Geometry check sheet. Reference: the model listing, model coordinates, mm. Face numbers are marked on the shaded views. A direction names the side the tool comes from. Give positions to 0.01 mm unless a question says otherwise; leave off trailing zeros. Loops run counter-clockwise (first coordinate to the right, second up) from the corner with the lowest first, then second, coordinate; pieces in that order, holes last. Notation, with made-up numbers: (80.25, 80) -> (109.25, 80) arc R14 cw to (109.25, 97) -> close; hole circle Ø4 at (-26, 5.25). An arc over 180 degrees is marked (long way). Write each question's results on one line, items separated by ' | '. Start each with the question number.
1) Sectioned sample at B-B on x = -28. Record the cut outline in (y, z).
2) Set-up check for the marked faces 4, 5 and 6: record each of +Z, -Z, +X, -X, +Y, -Y from which the full face is reachable in a straight line by a thin tool's end or side.
3) Draft check along Y on the marked faces 1, 2 and 3. Enter one of: pulls with the +Y half, pulls with the -Y half, needs draft (parallel to the pull), parting line crosses it, or undercut.
4) Scan lines: line 1 (X direction, y = 1, z = 0); line 2 (Y direction, x = -18.5, z = -38); line 3 (Y direction, x = -21.5, z = -37). Record each from-to range of solid material in increasing order. Write a range as from..to.
5) Sectioned sample at D-D on y = -30.5. Record the cut outline in (x, z), then the cut area to 3 significant figures.
6) Sectioned sample at A-A on z = 0. Record the cut outline in (x, y), then the cut area to 3 significant figures.
7) Sectioned sample at C-C on x = 5.08. Record the cut outline in (y, z), then the cut area to 3 significant figures.
8) Depth check by flat-ended pin: pin 1 (5 mm diameter, centred on y = 59, z = -19, fed in from -X); pin 2 (3 mm diameter, centred on y = 13.5, z = -20.5, fed in from +X); pin 3 (1 mm diameter, centred on y = 13, z = -44, fed in from +X). Enter the tip coordinate at first touch or a pass-through.
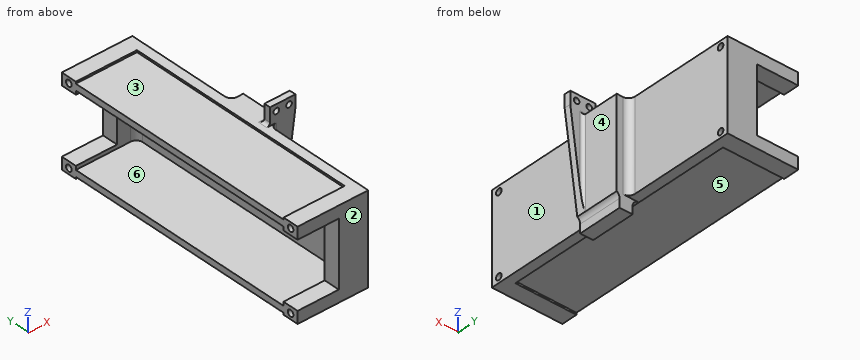
```python
from build123d import *

# Parameters (mm, degrees)
SKETCH1_R           = 1.1303
BOSS_EXTRUDE1_DEPTH = 2.54
SKETCH2_W           = 5.08
SKETCH2_H           = 35.814
BOSS_EXTRUDE2_DEPTH = 15.24
SKETCH3_W           = 35.814
SKETCH3_H           = 106.370628
BOSS_EXTRUDE3_DEPTH = 3.81
FILLET1_R           = 1.27
SKETCH4_W           = 5.191
SKETCH4_H           = 17.78
BOSS_EXTRUDE4_DEPTH = 5.588
SKETCH5_W           = 35.814
SKETCH5_H           = 6.35
BOSS_EXTRUDE5_DEPTH = 7.9756
SKETCH6_W           = 4.826
SKETCH6_H           = 6.35
BOSS_EXTRUDE6_DEPTH = 16.51
BOSS_EXTRUDE8_START = -0.762
SKETCH7_W           = 24.4856
SKETCH7_H           = 93.670628
BOSS_EXTRUDE8_DEPTH = 2.54
FILLET2_R           = 2.54
SKETCH8_R           = 1.27
CUT_EXTRUDE1_DEPTH  = 87.153909833


with BuildPart() as part:
    # Sketch1 → Boss-Extrude1 (new body)
    with BuildSketch(Plane(origin=(0, 0, 0), x_dir=(1, 0, 0), z_dir=(0, 1, 0))):
        Polygon((-2.54, 2.54), (-2.54, 40.132), (2.54, 40.132), (7.62, 2.54), (7.62, -2.54), (-2.54, -2.54), align=None)
        with Locations(Location((0, 0, 0), (0, 0, 270))):
            Circle(SKETCH1_R, mode=Mode.SUBTRACT)
        with Locations(Location((5.08, 0, 0), (0, 0, 270))):
            Circle(SKETCH1_R, mode=Mode.SUBTRACT)
    extrude(amount=BOSS_EXTRUDE1_DEPTH)

    # Sketch2 → Boss-Extrude2 (add)
    with BuildSketch(Plane(origin=(0, 2.54, 0), x_dir=(1, 0, 0), z_dir=(0, 1, 0))):
        with Locations((0, 22.225)):
            Rectangle(SKETCH2_W, SKETCH2_H)
    extrude(amount=BOSS_EXTRUDE2_DEPTH)

    # Sketch3 → Boss-Extrude3 (add)
    with BuildSketch(Plane.ZY.offset(2.54)):
        with Locations((-22.225, 8.89)):
            Rectangle(SKETCH3_W, SKETCH3_H)
    extrude(amount=BOSS_EXTRUDE3_DEPTH)

    # Fillet1
    fillet1_edges = [part.edges().sort_by_distance(p)[0] for p in [
        (0, 2.54, -4.318),
        (2.54, 2.54, -22.225),
        (-2.54, 1.27, -4.318),
    ]]
    fillet(fillet1_edges, radius=FILLET1_R)

    # Sketch4 → Boss-Extrude4 (add)
    with BuildSketch(Plane(origin=(0, 0, -40.132), x_dir=(-1, 0, 0), z_dir=(0, 0, -1))):
        with Locations((1.2145, 8.89)):
            Rectangle(SKETCH4_W, SKETCH4_H)
    extrude(amount=BOSS_EXTRUDE4_DEPTH)

    # Sketch5 → Boss-Extrude5 (add)
    with BuildSketch(Plane.ZY.offset(6.35)):
        with Locations((-22.225, -41.120314)):
            Rectangle(SKETCH5_W, SKETCH5_H)
        with Locations((-22.225, 58.900314)):
            Rectangle(SKETCH5_W, SKETCH5_H)
    extrude(amount=BOSS_EXTRUDE5_DEPTH)

    # Sketch6 → Boss-Extrude6 (add)
    with BuildSketch(Plane.ZY.offset(14.3256)):
        with Locations((-37.719, 58.900314)):
            Rectangle(SKETCH6_W, SKETCH6_H)
        with Locations((-6.731, 58.900314)):
            Rectangle(SKETCH6_W, SKETCH6_H)
        with Locations((-37.719, -41.120314)):
            Rectangle(SKETCH6_W, SKETCH6_H)
        with Locations((-6.731, -41.120314)):
            Rectangle(SKETCH6_W, SKETCH6_H)
    extrude(amount=BOSS_EXTRUDE6_DEPTH)

    # Sketch7 → Boss-Extrude8 (add)
    with BuildSketch(Plane.XY.offset(-4.318).offset(BOSS_EXTRUDE8_START)):
        with Locations((-18.5928, 8.89)):
            Rectangle(SKETCH7_W, SKETCH7_H)
    boss_extrude8 = extrude(amount=-BOSS_EXTRUDE8_DEPTH)

    # Mirror2: Boss-Extrude8 across plane
    add(boss_extrude8.mirror(Plane.XY.offset(-22.225)))

    # Fillet2
    # the kernel refuses this fillet: 2.54 mm, written as the material it adds along each edge
    with BuildSketch(Plane(origin=(-6.35, -37.945314, -1.27), x_dir=(-1, 0, 0), z_dir=(0, 0, -1))) as fillet2_piece_1_section:
        with BuildLine():
            CenterArc((FILLET2_R, FILLET2_R), FILLET2_R, 180, 90)
            Line((0, FILLET2_R), (0, 0))
            Line((0, 0), (FILLET2_R, 0))
        make_face()
    fillet2_piece_1 = extrude(amount=35.56, mode=Mode.PRIVATE)
    fillet2_piece_1 = split(fillet2_piece_1, bisect_by=Plane(origin=(-6.917354565, -37.377959435, -5.08), z_dir=(0, 0, -1)), keep=Keep.TOP, mode=Mode.PRIVATE)
    add(fillet2_piece_1)
    with BuildSketch(Plane(origin=(-6.35, 55.725314, -36.83), x_dir=(-1, 0, 0), z_dir=(0, 0, 1))) as fillet2_piece_2_section:
        with BuildLine():
            CenterArc((FILLET2_R, FILLET2_R), FILLET2_R, 180, 90)
            Line((0, FILLET2_R), (0, 0))
            Line((0, 0), (FILLET2_R, 0))
        make_face()
    fillet2_piece_2 = extrude(amount=35.56, mode=Mode.PRIVATE)
    fillet2_piece_2 = split(fillet2_piece_2, bisect_by=Plane(origin=(-6.917354565, 55.157959435, -5.08), z_dir=(0, 0, -1)), keep=Keep.TOP, mode=Mode.PRIVATE)
    add(fillet2_piece_2)
    with BuildSketch(Plane(origin=(-2.54, 17.78, -4.318), x_dir=(1, 0, 0), z_dir=(0, 0, -1)), Plane(origin=(-2.54, 0, -40.132), x_dir=(1, 0, 0), z_dir=(0, 0, 1))) as fillet2_piece_3:
        with BuildLine():
            CenterArc((FILLET2_R, -FILLET2_R), FILLET2_R, 90, 90)
            Line((0, -FILLET2_R), (0, 0))
            Line((0, 0), (FILLET2_R, 0))
        make_face()
    extrude(amount=35.814)
    with BuildSketch(Plane(origin=(1.381, 0, -40.132), x_dir=(0, 0, -1), z_dir=(0, 1, 0))) as fillet2_piece_4:
        with BuildLine():
            CenterArc((2.131768984, -2.54), FILLET2_R, 90, 57.064075369)
            Line((0, -1.159), (0, 0))
            Line((0, 0), (2.131768984, 0))
        make_face()
    extrude(amount=3.810000082)
    with BuildSketch(Plane(origin=(1.381, 3.810000082, -40.132), x_dir=(0, 0, -1), z_dir=(0, 1, 0))) as fillet2_piece_5:
        with BuildLine():
            CenterArc((2.131768984, -2.54), FILLET2_R, 90, 57.064075369)
            Line((0, -1.159), (0, 0))
            Line((0, 0), (2.131768984, 0))
        make_face()
    extrude(amount=13.969999918)
    with BuildSketch(Plane(origin=(-3.81, 17.78, -40.132), x_dir=(-1, 0, 0), z_dir=(0, -1, 0))) as fillet2_piece_6:
        with BuildLine():
            CenterArc((FILLET2_R, FILLET2_R), FILLET2_R, 180, 90)
            Line((0, FILLET2_R), (0, 0))
            Line((0, 0), (FILLET2_R, 0))
        make_face()
    extrude(amount=17.78)

    # Sketch8 → Cut-Extrude1 (cut, through all)
    with BuildSketch(Plane.ZY.offset(30.8356)):
        with Locations((-37.846, 58.900314)):
            Circle(SKETCH8_R)
        with Locations((-6.604, 58.900314)):
            Circle(SKETCH8_R)
        with Locations((-37.846, -41.120314)):
            Circle(SKETCH8_R)
        with Locations((-6.604, -41.120314)):
            Circle(SKETCH8_R)
    extrude(amount=-CUT_EXTRUDE1_DEPTH, mode=Mode.SUBTRACT)


solid = part.part
```
Result:
1) outline: (-44.3, -40.13) -> (-37.95, -40.13) -> (-37.95, -39.37) -> (55.73, -39.37) -> (55.73, -40.13) -> (62.08, -40.13) -> (62.08, -35.31) -> (55.73, -35.31) -> (55.73, -36.83) -> (-37.95, -36.83) -> (-37.95, -35.31) -> (-44.3, -35.31) -> close; (-44.3, -9.14) -> (-37.95, -9.14) -> (-37.95, -7.62) -> (55.73, -7.62) -> (55.73, -9.14) -> (62.08, -9.14) -> (62.08, -4.32) -> (55.73, -4.32) -> (55.73, -5.08) -> (-37.95, -5.08) -> (-37.95, -4.32) -> (-44.3, -4.32) -> close; hole circle Ø2.54 at (-41.12, -37.85); hole circle Ø2.54 at (-41.12, -6.6); hole circle Ø2.54 at (58.9, -37.85); hole circle Ø2.54 at (58.9, -6.6)
2) face 4: +Z, -Z, +X, +Y | face 5: -Z, -X | face 6: -X
3) face 1: needs draft | face 2: pulls with the -Y half | face 3: undercut
4) line 1: -2.54..-1.13, 1.13..3.95, 6.21..7.62 | line 2: -44.3..-42.38, -39.86..57.64, 60.16..62.08 | line 3: -44.3..-42.07, -40.17..57.95, 59.85..62.08
5) outline: (-30.84, -39.37) -> (-6.35, -39.37) -> (-6.35, -40.13) -> (-2.54, -40.13) -> (-2.54, -4.32) -> (-6.35, -4.32) -> (-6.35, -5.08) -> (-30.84, -5.08) -> (-30.84, -7.62) -> (-6.35, -7.62) -> (-6.35, -36.83) -> (-30.84, -36.83) -> close | area: 261 mm^2
6) outline: (-2.54, 0) -> (-1.13, 0) -> (-1.13, 2.54) -> (-2.54, 2.54) -> close; (1.13, 0) -> (3.95, 0) -> (3.95, 2.54) -> (1.13, 2.54) -> close; (6.21, 0) -> (7.62, 0) -> (7.62, 2.54) -> (6.21, 2.54) -> close | area: 14.3 mm^2
7) outline: (0, -21.34) -> (2.54, -21.34) -> (2.54, -1.13) -> (0, -1.13) -> close; (0, 1.13) -> (2.54, 1.13) -> (2.54, 2.54) -> (0, 2.54) -> close | area: 54.9 mm^2
8) pin 1: x = -14.33 | pin 2: x = 2.54 | pin 3: x = 1.38
